CAD build for the part. Positions are in the model's coordinates, mm. A direction names the side the tool comes from. Round coordinates to 2 decimals unless told otherwise and drop trailing zeros. Order: outer loops, then holes, each group sorted by start corner. A loop starts at its lowest first (then second) coordinate and runs counter-clockwise, first axis right, second up. Notation, with made-up numbers: (55.25, -18) -> (94.25, -18) arc R20 ccw to (94.25, 4) -> close; hole circle Ø7 at (-15, 42). An arc over 180 degrees is marked (long way). Return JSON: item names as keys, results as strings. Group by question number.
Q1. Cut at C-C (z = -21). Write the cut outline in (x, y).
Q2. Probe line 1 along Y through (x, z) = (86, -11); line 2 along Z through (x, y) = (66, -12); line 3 along Z through (x, y) = (82.5, 4.5). List the from-to ranges inside material, lowest first.
Q3. Cut at A-A (y = -40.5). Write the cut outline in (x, z), then the cut area to 3 significant figures.
Q4. Which spindle directions (+Z, -Z, +X, -X, +Y, -Y) get a long thin tool onto all of the face, cutting with end or side? Do faces 1 (the flat face through (70.994, -42, 30)), 2 (the flat face through (42.725, 6.409, -2.651)), 3 (the cylindrical face through (98.599, 6.639, 14.322)), 4 (the cylindrical face through (37.99, 5.35, 13.94)). Say none if no direction does.
Q5. Flat gauge pins, fed straight in: pin 1 (8 mm diameter, centred on y = -36, z = 26.5, fed in from +X); pin 2 (3.5 mm diameter, centred on y = -7, z = 29.5, fed in from +X); pin 3 (5 mm diameter, centred on y = 6.5, z = 11.17, fed in from -X); pin 4 (2 mm diameter, centred on y = 1, z = 10, fed in from -X). Where does each tip first touch, or does it go through?
Q6. Mould opens along Z. For faces 5 (the flat face through (67, -40, 24.392)), 6 (the flat face through (44, 13, 11)), 7 (the flat face through (94.83, 6.41, 2.75)) say: +Z half, -Z half, draft (parallel to the pull), parting line (faces both ways), or undercut.
Q7. Cut at D-D (z = -13). Count the separate pieces of the cut face and the enclosed holes in it, then the cut area to 3 significant figures.
Q8. Cut at B-B (x = 75.5). Write the cut outline in (y, z), then the cut area to 3 significant figures.
from build123d import *

# Parameters (mm, degrees)
BOSS_EXTRUDE1_DEPTH      = 13
SKETCH4_W                = 8
SKETCH4_H                = 2
BOSS_EXTRUDE2_DEPTH      = 43
SKETCH5_W                = 8
SKETCH5_H                = 5
BOSS_EXTRUDE3_DEPTH      = 12
SKETCH6_R                = 1
CUT_EXTRUDE3_DEPTH       = 13
FILLET1_R                = 10
BOSS_EXTRUDE4_DEPTH      = 2
SKETCH11_R               = 37.7
BOSS_EXTRUDE5_DEPTH      = 13
SKETCH22_R               = 1.25
CUT_EXTRUDE6_DEPTH       = 83
SKETCH22_3_R             = 3.155829002
SKETCH22_3_R_2           = 1.25
CUT_EXTRUDE7_DEPTH       = 15
SKETCH23_R               = 3
CUT_EXTRUDE8_DEPTH       = 15
BOSS_EXTRUDE6_REACH      = 133.524
BOSS_EXTRUDE6_END_RADIUS = 37.7
SKETCH26_R               = 2
CUT_EXTRUDE9_DEPTH       = 88
SKETCH27_R               = 2
CUT_EXTRUDE10_DEPTH      = 120
SKETCH28_W               = 5.884393281
SKETCH28_H               = 23.801066831
CUT_EXTRUDE11_DEPTH      = 2.5
CUT_EXTRUDE12_REACH      = 126.386


with BuildPart() as part:
    # Sketch2 → Boss-Extrude1 (new body)
    with BuildSketch(Plane(origin=(0, 0, 0), x_dir=(1, 0, 0), z_dir=(0, 1, 0))):
        Polygon((56.165444193, 16.052878064), (80.422298442, 16.052878064), (87.816410992, 8.658765514), (87.816410992, -30.998088735), (80.422298442, -38.392201285), (56.165444193, -38.392201285), (48.771331643, -30.998088735), (48.771331643, 8.658765514), align=None)
        Polygon((50.771331643, -30.16966161), (50.771331643, 7.83033839), (56.993871317, 14.052878064), (79.593871317, 14.052878064), (85.816410992, 7.83033839), (85.816410992, -30.16966161), (79.593871317, -36.392201285), (56.993871317, -36.392201285), align=None, mode=Mode.SUBTRACT)
    extrude(amount=BOSS_EXTRUDE1_DEPTH)

    # Sketch4 → Boss-Extrude2 (add)
    with BuildSketch(Plane.XZ):
        with Locations((66.993871317, 37.392201285)):
            Rectangle(SKETCH4_W, SKETCH4_H)
    extrude(amount=BOSS_EXTRUDE2_DEPTH)

    # Sketch5 → Boss-Extrude3 (add)
    with BuildSketch(Plane(origin=(0, 0, 36.392201285), x_dir=(-1, 0, 0), z_dir=(0, 0, -1))):
        with Locations((-66.993871317, -12.5)):
            Rectangle(SKETCH5_W, SKETCH5_H)
        with Locations((-66.993871317, -40.5)):
            Rectangle(SKETCH5_W, SKETCH5_H)
    extrude(amount=BOSS_EXTRUDE3_DEPTH)

    # Sketch6 → Cut-Extrude3 (cut)
    with BuildSketch(Plane.ZY.offset(-62.993871317)):
        with Locations((30.392201285, -12.5)):
            Circle(SKETCH6_R)
        with Locations((30.392201285, -40.5)):
            Circle(SKETCH6_R)
    extrude(amount=-CUT_EXTRUDE3_DEPTH, mode=Mode.SUBTRACT)

    # Fillet1
    fillet1_edges = [part.edges().sort_by_distance(p)[0] for p in [
        (66.993871317, -10, 36.392201285),
    ]]
    fillet(fillet1_edges, radius=FILLET1_R)

    # Sketch10 → Boss-Extrude4 (add)
    with BuildSketch(Plane.XY.offset(38.392201285)):
        Polygon((56.165444193, 0), (62.993871317, -43), (70.993871317, -43), (80.422298442, 0), align=None)
    extrude(amount=-BOSS_EXTRUDE4_DEPTH)

    # Sketch11 → Boss-Extrude5 (add)
    with BuildSketch(Plane(origin=(0, 13, 0), x_dir=(1, 0, 0), z_dir=(0, 1, 0))):
        with Locations(Location((68.293871317, -11.16966161, 0), (0, 0, 270))):
            Circle(SKETCH11_R)
        Polygon((56.165444193, 16.052878064), (48.771331643, 8.658765514), (48.771331643, -30.998088735), (56.165444193, -38.392201285), (80.422298442, -38.392201285), (87.816410992, -30.998088735), (87.816410992, 8.658765514), (80.422298442, 16.052878064), align=None, mode=Mode.SUBTRACT)
    extrude(amount=-BOSS_EXTRUDE5_DEPTH)

    # Sketch22 → Cut-Extrude6 (cut)
    with BuildSketch(Plane(origin=(105.993871317, 0, 0), x_dir=(0, 0, -1), z_dir=(1, 0, 0))):
        with Locations((-11.16966161, 6.5)):
            Circle(SKETCH22_R)
    extrude(amount=-CUT_EXTRUDE6_DEPTH, mode=Mode.SUBTRACT)

    # Sketch22<3> → Cut-Extrude7 (cut)
    with BuildSketch(Plane(origin=(105.993871317, 0, 0), x_dir=(0, 0, -1), z_dir=(1, 0, 0))):
        with Locations((-11.16966161, 6.5)):
            Circle(SKETCH22_3_R)
        with Locations((-11.16966161, 6.5)):
            Circle(SKETCH22_3_R_2, mode=Mode.SUBTRACT)
    extrude(amount=-CUT_EXTRUDE7_DEPTH, mode=Mode.SUBTRACT)

    # Sketch23 → Cut-Extrude8 (cut)
    with BuildSketch(Plane.ZY.offset(-30.593871317)):
        with Locations((11.16966161, 6.5)):
            Circle(SKETCH23_R)
    extrude(amount=-CUT_EXTRUDE8_DEPTH, mode=Mode.SUBTRACT)

    # Boss-Extrude6: up to this cylinder (the profile starts inside it)
    boss_extrude6_end = Plane(origin=(68.293871317, -17.888133, 11.16966161), z_dir=(0, 1, 0)) * Cylinder(BOSS_EXTRUDE6_END_RADIUS, 343.448, mode=Mode.PRIVATE)
    # Sketch25 → Boss-Extrude6 (add, up to the surface)
    with BuildSketch(Plane.XY.offset(38.392201285), mode=Mode.PRIVATE) as boss_extrude6_sk1:
        Polygon((80.422298442, 0), (56.165444193, 0), (62.993871317, -43), (70.993871317, -43), align=None)
    boss_extrude6_tool1 = extrude(boss_extrude6_sk1.sketch, amount=BOSS_EXTRUDE6_REACH, mode=Mode.PRIVATE) & boss_extrude6_end
    add(boss_extrude6_tool1.solids().sort_by_distance((67.753067, -17.888133, 38.392201))[0])

    # Sketch26 → Cut-Extrude9 (cut)
    with BuildSketch(Plane(origin=(1.904179203, 0, -1.904179203), x_dir=(0.7071067811865485, 0, 0.7071067811865467), z_dir=(-0.7071067811865467, 0, 0.7071067811865485))):
        with Locations((56.18920299, 6.5)):
            Circle(SKETCH26_R)
    extrude(amount=-CUT_EXTRUDE9_DEPTH, mode=Mode.SUBTRACT)

    # Sketch27 → Cut-Extrude10 (cut)
    with BuildSketch(Plane(origin=(66.389692115, 0, 66.389692115), x_dir=(0.7071067811865477, 0, -0.7071067811865474), z_dir=(0.7071067811865474, 0, 0.7071067811865477))):
        with Locations((40.392916054, 6.5)):
            Circle(SKETCH27_R)
    extrude(amount=-CUT_EXTRUDE10_DEPTH, mode=Mode.SUBTRACT)

    # Sketch28 → Cut-Extrude11 (cut)
    with BuildSketch(Plane.XZ):
        with Locations((88.758607633, 11.900533415)):
            Rectangle(SKETCH28_W, SKETCH28_H)
    extrude(amount=-CUT_EXTRUDE11_DEPTH, mode=Mode.SUBTRACT)

    # Sketch30 → Cut-Extrude12 (cut, up to next)
    with BuildSketch(Plane.XZ, mode=Mode.PRIVATE) as cut_extrude12_sk1:
        with BuildLine():
            Line((50.771331643, -7.83033839), (85.816410992, -7.83033839))
            ThreePointArc((85.816410992, -7.83033839), (68.293871317, -22.826628819), (50.771331643, -7.83033839))
        make_face()
    cut_extrude12_tool1 = extrude(cut_extrude12_sk1.sketch, amount=-CUT_EXTRUDE12_REACH, mode=Mode.PRIVATE) & part.part
    # Sketch30 → Cut-Extrude12 (cut, up to next)
    with BuildSketch(Plane.XZ, mode=Mode.PRIVATE) as cut_extrude12_sk2:
        Polygon((38.741691169, -7.83033839), (34.266383325, 2.385887147), (46.597716142, 2.385887147), align=None)
    cut_extrude12_tool2 = extrude(cut_extrude12_sk2.sketch, amount=-CUT_EXTRUDE12_REACH, mode=Mode.PRIVATE) & part.part
    # Sketch30 → Cut-Extrude12 (cut, up to next)
    with BuildSketch(Plane.XZ, mode=Mode.PRIVATE) as cut_extrude12_sk3:
        Polygon((97.389775461, -7.83033839), (87.532944471, 0), (102.33223512, 5.578425036), align=None)
    cut_extrude12_tool3 = extrude(cut_extrude12_sk3.sketch, amount=-CUT_EXTRUDE12_REACH, mode=Mode.PRIVATE) & part.part
    # Sketch30 → Cut-Extrude12 (cut, up to next)
    with BuildSketch(Plane.XZ, mode=Mode.PRIVATE) as cut_extrude12_sk4:
        Polygon((102.33223512, 18.629349006), (88.758607633, 23.801066831), (95.998995796, 32.915268399), align=None)
    cut_extrude12_tool4 = extrude(cut_extrude12_sk4.sketch, amount=-CUT_EXTRUDE12_REACH, mode=Mode.PRIVATE) & part.part
    # Sketch30 → Cut-Extrude12 (cut, up to next)
    with BuildSketch(Plane.XZ, mode=Mode.PRIVATE) as cut_extrude12_sk5:
        Polygon((34.266383325, 18.629349006), (38.741691169, 31.410722253), (46.597716142, 23.801066831), align=None)
    cut_extrude12_tool5 = extrude(cut_extrude12_sk5.sketch, amount=-CUT_EXTRUDE12_REACH, mode=Mode.PRIVATE) & part.part
    add(cut_extrude12_tool1.solids().sort_by_distance((68.293871, 0, -14.118791))[0], mode=Mode.SUBTRACT)
    add(cut_extrude12_tool2.solids().sort_by_distance((39.868597, 0, -1.019521))[0], mode=Mode.SUBTRACT)
    add(cut_extrude12_tool3.solids().sort_by_distance((95.751652, 0, -0.750638))[0], mode=Mode.SUBTRACT)
    add(cut_extrude12_tool4.solids().sort_by_distance((95.696613, 0, 25.115228))[0], mode=Mode.SUBTRACT)
    add(cut_extrude12_tool5.solids().sort_by_distance((39.868597, 0, 24.613713))[0], mode=Mode.SUBTRACT)


solid = part.part
Solution:
{
 "1": {"outline": "(48.64, 0) -> (60.45, 0) -> (60.45, 13) -> (48.64, 13) -> close; (76.13, 0) -> (87.95, 0) -> (87.95, 13) -> (76.13, 13) -> close"},
 "2": {"line 1": "y = 0 to 13", "line 2": "z = 24.39 to 29.53, 31.26 to 48.8", "line 3": "z = -23.75 to -15.71, 33.49 to 46.09"},
 "3": {"outline": "(62.6, 36.39) -> (62.99, 36.39) -> (62.99, 31.39) -> (70.99, 31.39) -> (70.99, 36.39) -> (71.54, 36.39) -> (71.54, 48.73) arc R37.7 ccw to (62.6, 48.44) -> close; (62.99, 24.39) -> (70.99, 24.39) -> (70.99, 29.39) -> (62.99, 29.39) -> close", "area": "191 mm²"},
 "4": {"face 1": "-Z, +X, +Y, -Y", "face 2": "+Y, -Y", "face 3": "+X", "face 4": "-X"},
 "5": {"pin 1": "stops at x = 70.99", "pin 2": "passes through", "pin 3": "stops at x = 45.59", "pin 4": "stops at x = 30.59"},
 "6": {"face 5": "-Z half", "face 6": "draft", "face 7": "undercut"},
 "7": {"separate pieces": "2", "enclosed holes": "2", "area": "304 mm²"},
 "8": {"outline": "(-22.45, 36.39) -> (13, 36.39) -> (13, 48.17) -> (-22.45, 48.17) -> close; (0, -25.84) -> (13, -25.84) -> (13, -21.3) -> (0, -21.3) -> close", "area": "477 mm²"}
}
